Read the model definition and answer for the solid it produces. Units are mm, in the model's axes. A direction names the side the tool comes from. Round coordinates to 2 decimals unless told otherwise and drop trailing zeros. Write each loop counter-clockwise with the first axis right and the second up, starting at its lowest first coordinate (ties: lowest second). Pieces come first, ordered by that corner, then holes. Notation, with made-up numbers: (60.25, 58.5) - (95.25, 58.5) arc R26 cw to (95.25, 92.5) - close; hole circle Ø1 at (53, 45.25). An arc over 180 degrees is marked (long way). Answer as CSV lines item,"result". Start each with the question number.
1) Consider line 1 along X through (y, z) = (732, -143); line 2 along Y through (x, z) = (55, 18.5); line 3 along Z through (x, y) = (80.5, 75). Determine where each line is inside the solid, lowest interval first.
2) Find section D-D on x = 67. Determine the outline of the cut face in (y, z).
3) Find section A-A on y = 773. Determine the outline of the cut face in (x, z).
4) For a pull along Y with two mould halves and no side action, classify faces 1 (the flat face through (19, 807, -210)), 2 (the flat face through (-480.513, 140.601, -154.79)), 3 (the flat face through (-225, 141, 127)) as +Y half, -Y half, draft (parallel to the pull), parting line (faces both ways), or undercut.
5) Find section B-B on y = 266. Determine the outline of the cut face in (x, z), then the cut area to 3 significant figures.
6) Each of these flat-tipped pins is pushed along its axis until it touches: pin 1 (4 mm diameter, centred on x = -465, z = 107.5, fed in from +Y); pin 2 (6 mm diameter, centred on y = 551, z = 9.5, fed in from +X); pin 3 (1.5 mm diameter, centred on y = 837.5, z = -178.5, fed in from -X). Where does it stop, or does it pass through?
7) Find section C-C on z = 68. Determine the outline of the cut face in (x, y).
8) Which of the six approach directions +Z, -Z, +X, -X, +Y, -Y give full straight-line access (tool end or side, diameter ignored) to faces 4 (the flat face through (34, 624, -252.5)), 5 (the flat face through (140, 980, 4)), 6 (the flat face through (-54.617, 170.139, 111.79))?
from build123d import *

# Parameters (mm, degrees)
BOSS_EXTRUDE1_DEPTH  = 40
SKETCH3_W            = 505
SKETCH3_H            = 30
BOSS_EXTRUDE2_DEPTH  = 100
BOSS_EXTRUDE3_START  = 205
SKETCH5_R            = 100
BOSS_EXTRUDE3_DEPTH  = 75
BOSS_EXTRUDE4_START  = -205
SKETCH5_2_R          = 100
BOSS_EXTRUDE4_DEPTH  = 75
SKETCH7_W            = 505
SKETCH7_H            = 381
BOSS_EXTRUDE5_DEPTH  = 30
SKETCH8_W            = 230
SKETCH8_H            = 440
SKETCH8_W_2          = 210
SKETCH8_H_2          = 420
EXTRUDE_THIN1_DEPTH  = 210
SKETCH9_W            = 230
SKETCH9_H            = 440
BOSS_EXTRUDE6_DEPTH  = 10
SKETCH10_W           = 505
SKETCH10_H           = 7.5
BOSS_EXTRUDE7_DEPTH  = 7.5
BOSS_EXTRUDE8_START  = 205
BOSS_EXTRUDE8_DEPTH  = 15
BOSS_EXTRUDE9_START  = -205
BOSS_EXTRUDE9_DEPTH  = 15
BOSS_EXTRUDE10_REACH = 1238.243
SKETCH12_W           = 44.047720934
SKETCH12_H           = 61.152550191
BOSS_EXTRUDE11_START = 140
SKETCH13_R           = 62.5
BOSS_EXTRUDE11_DEPTH = 30
BOSS_EXTRUDE12_START = -140
SKETCH13_4_R         = 62.5
BOSS_EXTRUDE12_DEPTH = 30
EXTRUDE_THIN5_DEPTH  = 15
LPATTERN1_COUNT      = 2
LPATTERN1_PITCH      = 112
SKETCH15_W           = 7.5
SKETCH15_H           = 7.5
CUT_EXTRUDE1_DEPTH   = 60
MIRROR1_COPY_1_DEPTH = 15
MIRROR1_COPY_2_DEPTH = 15


with BuildPart() as part:
    # Sketch1 → Boss-Extrude1 (new body)
    with BuildSketch(Plane(origin=(0, 0, 0), x_dir=(0, 0, -1), z_dir=(1, 0, 0))):
        Polygon((-232.5, 0), (-252.5, 0), (-252.5, 995), (252.5, 995), (252.5, 0), (232.5, 0), (232.5, 965), (-232.5, 965), align=None)
    extrude(amount=BOSS_EXTRUDE1_DEPTH)

    # Sketch3 → Boss-Extrude2 (add)
    with BuildSketch(Plane(origin=(40, 0, 0), x_dir=(0, 0, -1), z_dir=(1, 0, 0))):
        with Locations((0, 980)):
            Rectangle(SKETCH3_W, SKETCH3_H)
    extrude(amount=BOSS_EXTRUDE2_DEPTH)

    # Sketch5<2> → Boss-Extrude4 (add)
    with BuildSketch(Plane.XY.offset(BOSS_EXTRUDE4_START)):
        with Locations((20, 100)):
            Circle(SKETCH5_2_R)
    extrude(amount=-BOSS_EXTRUDE4_DEPTH)

    # Sketch7 → Boss-Extrude5 (add)
    with BuildSketch(Plane(origin=(40, 0, 0), x_dir=(0, 0, -1), z_dir=(1, 0, 0))):
        with Locations((0, 507.5)):
            Rectangle(SKETCH7_W, SKETCH7_H)
    extrude(amount=-BOSS_EXTRUDE5_DEPTH)

    # Sketch8 → Extrude-Thin1 (add)
    with BuildSketch(Plane(origin=(0, 698, 0), x_dir=(1, 0, 0), z_dir=(0, 1, 0))):
        with Locations((20, 0)):
            Rectangle(SKETCH8_W, SKETCH8_H)
        with Locations((20, 0)):
            Rectangle(SKETCH8_W_2, SKETCH8_H_2, mode=Mode.SUBTRACT)
    extrude(amount=EXTRUDE_THIN1_DEPTH)

    # Sketch9 → Boss-Extrude6 (add)
    with BuildSketch(Plane.XZ.offset(-698)):
        with Locations((20, 0)):
            Rectangle(SKETCH9_W, SKETCH9_H)
    extrude(amount=-BOSS_EXTRUDE6_DEPTH)

    # Sketch10 → Boss-Extrude7 (add)
    with BuildSketch(Plane.ZY):
        with Locations((0, 236.25)):
            Rectangle(SKETCH10_W, SKETCH10_H)
    extrude(amount=BOSS_EXTRUDE7_DEPTH)


with BuildPart() as body_2:
    # Sketch5 → Boss-Extrude3 (new body)
    with BuildSketch(Plane.XY.offset(BOSS_EXTRUDE3_START)):
        with Locations((20, 100)):
            Circle(SKETCH5_R)
    extrude(amount=BOSS_EXTRUDE3_DEPTH)


    add(part.part)  # Boss-Extrude8 merges part
    # Sketch11 → Boss-Extrude8 (add)
    with BuildSketch(Plane.XY.offset(BOSS_EXTRUDE8_START)):
        Polygon((21.910116732, 109.815877652), (-533.089883268, 217.815877652), (-536.910116732, 198.184122348), (18.089883268, 90.184122348), align=None)
    extrude(amount=BOSS_EXTRUDE8_DEPTH)

    # Sketch11<2> → Boss-Extrude9 (add)
    with BuildSketch(Plane.XY.offset(BOSS_EXTRUDE9_START)):
        Polygon((21.910116732, 109.815877652), (-533.089883268, 217.815877652), (-536.910116732, 198.184122348), (18.089883268, 90.184122348), align=None)
    extrude(amount=-BOSS_EXTRUDE9_DEPTH)

    # Boss-Extrude10: up to this face of the body (flat: up to its plane)
    boss_extrude10_end = Plane(body_2.part.faces().sort_by_distance((-306.497442612, 163.534637481, -220))[0])
    # Sketch12 → Boss-Extrude10 (add, up to the picked face)
    with BuildSketch(Plane.XY.offset(220), mode=Mode.PRIVATE) as boss_extrude10_sk1:
        with Locations((-511.066022801, 187.239602557)):
            Rectangle(SKETCH12_W, SKETCH12_H)
    boss_extrude10_tool1 = split(extrude(boss_extrude10_sk1.sketch, amount=-BOSS_EXTRUDE10_REACH, mode=Mode.PRIVATE), bisect_by=boss_extrude10_end, keep=Keep.BOTH, mode=Mode.PRIVATE)
    add(boss_extrude10_tool1.solids().sort_by(Axis((-511.066023, 187.239603, 220), (0, 0, -1)))[0])

    # Sketch13 → Boss-Extrude11 (add)
    with BuildSketch(Plane.XY.offset(BOSS_EXTRUDE11_START)):
        with Locations((-461.066022801, 62.5)):
            Circle(SKETCH13_R)
        with BuildLine():
            Line((-493.886091971, 165.785738113), (-443.886091971, 71.622410652))
            ThreePointArc((-443.886091971, 71.622410652), (-451.943612148, 45.32006917), (-478.245953631, 53.377589348))
            Line((-478.245953631, 53.377589348), (-528.245953631, 147.540916809))
            ThreePointArc((-528.245953631, 147.540916809), (-520.188433453, 173.843258291), (-493.886091971, 165.785738113))
        make_face()
    extrude(amount=BOSS_EXTRUDE11_DEPTH)

    # Sketch13<4> → Boss-Extrude12 (add)
    with BuildSketch(Plane.XY.offset(BOSS_EXTRUDE12_START)):
        with Locations((-461.066022801, 62.5)):
            Circle(SKETCH13_4_R)
        with BuildLine():
            Line((-493.886091971, 165.785738113), (-443.886091971, 71.622410652))
            ThreePointArc((-443.886091971, 71.622410652), (-451.943612148, 45.32006917), (-478.245953631, 53.377589348))
            Line((-478.245953631, 53.377589348), (-528.245953631, 147.540916809))
            ThreePointArc((-528.245953631, 147.540916809), (-520.188433453, 173.843258291), (-493.886091971, 165.785738113))
        make_face()
    extrude(amount=-BOSS_EXTRUDE12_DEPTH)

    # Sketch14 → Extrude-Thin5 (add, symmetric)
    with BuildSketch(Plane.XY):
        Polygon((-7.52287052, 239.53107422), (-111.10842632, 120.419203046), (-488.087103968, 193.777215994), (-489.9972207, 183.961338343), (-107.351343448, 109.500518985), (0.02287052, 232.96892578), align=None)
    extrude_thin5 = extrude(amount=EXTRUDE_THIN5_DEPTH, both=True)

    # LPattern1: Extrude-Thin5 ×2
    with Locations(*[(0, 0, -i * LPATTERN1_PITCH) for i in range(1, LPATTERN1_COUNT)]):
        add(extrude_thin5)

    # Sketch15 → Cut-Extrude1 (cut)
    with BuildSketch(Plane(origin=(0, 0, -252.5), x_dir=(-1, 0, 0), z_dir=(0, 0, -1))):
        with Locations((3.75, 236.25)):
            Rectangle(SKETCH15_W, SKETCH15_H)
    cut_extrude1 = extrude(amount=-CUT_EXTRUDE1_DEPTH, mode=Mode.SUBTRACT)

    # Mirror1: Cut-Extrude1 across plane
    add(cut_extrude1.mirror(Plane.XY), mode=Mode.SUBTRACT)

    # Mirror1 copy 1 sketch → Mirror1 copy 1 (add, symmetric)
    with BuildSketch(Plane(origin=(0, 0, 112), x_dir=(1, 0, 0), z_dir=(0, 0, -1))):
        Polygon((-7.52287052, -239.53107422), (-111.10842632, -120.419203046), (-488.087103968, -193.777215994), (-489.9972207, -183.961338343), (-107.351343448, -109.500518985), (0.02287052, -232.96892578), align=None)
    extrude(amount=MIRROR1_COPY_1_DEPTH, both=True)

    # Mirror1 copy 2 sketch → Mirror1 copy 2 (add, symmetric)
    with BuildSketch(Plane(origin=(0, 0, 0), x_dir=(1, 0, 0), z_dir=(0, 0, -1))):
        Polygon((-7.52287052, -239.53107422), (-111.10842632, -120.419203046), (-488.087103968, -193.777215994), (-489.9972207, -183.961338343), (-107.351343448, -109.500518985), (0.02287052, -232.96892578), align=None)
    extrude(amount=MIRROR1_COPY_2_DEPTH, both=True)


solid = body_2.part
Check values:
1,line 1,"x = -95 to -85, 125 to 135"
1,line 2,"y = 698 to 708, 965 to 995"
1,line 3,"z = -280 to -205, 205 to 280"
2,outline,"(11.73, -280) - (188.27, -280) - (188.27, -205) - (11.73, -205) - close; (11.73, 205) - (188.27, 205) - (188.27, 280) - (11.73, 280) - close; (698, -220) - (908, -220) - (908, -210) - (708, -210) - (708, 210) - (908, 210) - (908, 220) - (698, 220) - close; (965, -252.5) - (995, -252.5) - (995, 252.5) - (965, 252.5) - close"
3,outline,"(-95, -220) - (135, -220) - (135, 220) - (-95, 220) - close; (0, -252.5) - (40, -252.5) - (40, -232.5) - (0, -232.5) - close; (0, 232.5) - (40, 232.5) - (40, 252.5) - (0, 252.5) - close; hole (-85, -210) - (125, -210) - (125, 210) - (-85, 210) - close"
4,face 1,"undercut"
4,face 2,"+Y half"
4,face 3,"draft"
5,outline,"(0, -252.5) - (40, -252.5) - (40, -232.5) - (0, -232.5) - close; (0, 232.5) - (40, 232.5) - (40, 252.5) - (0, 252.5) - close"
5,area,"1,600 mm^2"
6,pin 1,"stops at y = 189.67"
6,pin 2,"stops at x = 40"
6,pin 3,"stops at x = -95"
7,outline,"(-533.09, 156.66) - (-489.04, 156.66) - (-489.04, 217.82) - (-533.09, 217.82) - close; (-95, 698) - (10, 698) - (10, 317) - (40, 317) - (40, 698) - (135, 698) - (135, 908) - (125, 908) - (125, 708) - (-85, 708) - (-85, 908) - (-95, 908) - close; (-7.5, 232.5) - (0, 232.5) - (0, 240) - (-7.5, 240) - close; (0, 965) - (140, 965) - (140, 995) - (0, 995) - close"
8,face 4,"-Z, +X, -X, +Y"
8,face 5,"+Z, -Z, +X, +Y, -Y"
8,face 6,"+X, -Y"
